Could you check a few things on this model? Use its own coordinates, in mm. A direction names the side the tool comes from. Coordinates: 2 decimals unless noted, no trailing zeros. Loops run counter-clockwise (first coordinate to the right, second up) from the corner with the lowest first, then second, coordinate; pieces in that order, holes last. Notation, with made-up numbers: (38.5, -7) -> (70.5, -7) arc R19 ccw to (70.5, 0) -> close; hole circle Ø1 at (19, -33.75). An arc over 180 degrees is marked (long way). One line per question, with ' | ' between items. Start each with the question number.
(1) If I drill on line 1 along Y through (x, z) = (0, 3.45); line 2 along X through (y, z) = (-32, 2.5); line 3 along Y through (x, z) = (-0.5, 9.25), over which ranges is the centre line in solid material (lowest first)?
(2) If we mould it in two halves opening along Z, with no side actions, what happens to faces 4 (the face through (4.95, -42.93, 8.72)), 5 (the face through (-0.581, 47.317, 16.797)), 6 (the face through (0.434, 27.548, 2.465))? For each: pulls with the +Z half, pulls with the -Z half, needs draft (parallel to the pull), parting line crosses it, or undercut.
(3) I'm going to push flat-ended pins straight in: pin 1 Ø4 at (y, z) = (-31.5, 8.5) entering from +X; pin 2 Ø1.2 at (x, y) = (0, 29.5) entering from -Z; pin 3 Ø0.8 at (x, z) = (0, 8.5) entering from -Y. Where does each tip first touch, or does it pass through?
(4) Suppose I cut it at A-A (x = 0). Please give me the cut outline in (y, z), plus the area to 3 significant figures.
(5) Which directions (+Z, -Z, +X, -X, +Y, -Y) give clear straight access to the entire face, cutting with the end or side of a thin tool? Please do faces 1 (the face through (0, 30, 5)), 2 (the face through (-46.3, 20, 8)), 3 (the face through (0, -43, 7.47)).
```python
from build123d import *

# Parameters (mm, degrees)
SKETCH1_W           = 93
SKETCH1_H           = 97
BOSS_EXTRUDE1_DEPTH = 17.5
FILLET1_SIZE        = 5
FILLET1_SIZE_2      = 10
FILLET2_SIZE        = 10
FILLET2_SIZE_2      = 5
FILLET3_SIZE        = 5
FILLET3_SIZE_2      = 10
SKETCH2_R           = 1.28
SKETCH2_W           = 7.34
SKETCH2_H           = 2.56
CUT_EXTRUDE1_DEPTH  = 11.3
SKETCH3_R           = 5
BOSS_EXTRUDE2_DEPTH = 0.6
CHAMFER1_SIZE       = 0.6
CUT_EXTRUDE2_DEPTH  = 0.2
CHAMFER4_SIZE       = 2.4
CHAMFER4_SIZE2      = 1.385640646
SKETCH5_R           = 2
CUT_EXTRUDE3_DEPTH  = 5


# Some blends are built 0.0001 mm under size
with BuildPart() as part:
    # Sketch1 → Boss-Extrude1 (new body)
    with BuildSketch(Plane.XY):
        Rectangle(SKETCH1_W, SKETCH1_H)
    extrude(amount=BOSS_EXTRUDE1_DEPTH)

    # Fillet1
    # an asymmetric fillet: 10, 5 mm, written as the material it takes off along each edge
    with BuildSketch(Plane(origin=(-46.5, 48.5, -25), x_dir=(1, 0, 0), z_dir=(0, 0, 1))) as fillet1_piece_1:
        with BuildLine():
            Bezier((FILLET1_SIZE, 0), (0, 0), (0, -FILLET1_SIZE_2), weights=[1, 0.707106781, 1])
            Line((0, -FILLET1_SIZE_2), (0, 0))
            Line((0, 0), (FILLET1_SIZE, 0))
        make_face()
    extrude(amount=67.5, mode=Mode.SUBTRACT)
    with BuildSketch(Plane(origin=(46.5, -48.5, -25), x_dir=(0, 1, 0), z_dir=(0, 0, 1))) as fillet1_piece_2:
        with BuildLine():
            Bezier((FILLET1_SIZE_2, 0), (0, 0), (0, FILLET1_SIZE), weights=[1, 0.707106781, 1])
            Line((0, FILLET1_SIZE), (0, 0))
            Line((0, 0), (FILLET1_SIZE_2, 0))
        make_face()
    extrude(amount=67.5, mode=Mode.SUBTRACT)

    # Fillet2
    # an asymmetric fillet: 10, 5 mm, written as the material it takes off along each edge
    with BuildSketch(Plane(origin=(-46.5, -48.5, -25), x_dir=(0, 1, 0), z_dir=(0, 0, 1))) as fillet2_piece_1:
        with BuildLine():
            Bezier((FILLET2_SIZE, 0), (0, 0), (0, -FILLET2_SIZE_2), weights=[1, 0.707106781, 1])
            Line((0, -FILLET2_SIZE_2), (0, 0))
            Line((0, 0), (FILLET2_SIZE, 0))
        make_face()
    extrude(amount=67.5, mode=Mode.SUBTRACT)

    # Fillet3
    # an asymmetric fillet: 10, 5 mm, written as the material it takes off along each edge
    with BuildSketch(Plane(origin=(46.5, 48.5, -25), x_dir=(-1, 0, 0), z_dir=(0, 0, 1))) as fillet3_piece_1:
        with BuildLine():
            Bezier((FILLET3_SIZE, 0), (0, 0), (0, FILLET3_SIZE_2), weights=[1, 0.707106781, 1])
            Line((0, FILLET3_SIZE_2), (0, 0))
            Line((0, 0), (FILLET3_SIZE, 0))
        make_face()
    extrude(amount=67.5, mode=Mode.SUBTRACT)

    # Sketch2 → Cut-Extrude1 (cut)
    with BuildSketch(Plane.XZ.offset(48.5)):
        with Locations((-3.67, 8.75)):
            Circle(SKETCH2_R)
        with Locations((3.67, 8.75)):
            Circle(SKETCH2_R)
        with Locations((0, 8.75)):
            Rectangle(SKETCH2_W, SKETCH2_H)
    extrude(amount=-CUT_EXTRUDE1_DEPTH, mode=Mode.SUBTRACT)

    # Sketch3 → Boss-Extrude2 (add)
    with BuildSketch(Plane(origin=(46.5, 0, 0), x_dir=(0, 0, -1), z_dir=(1, 0, 0))):
        with Locations(Location((-7.7, 8.5, 0), (0, 0, 270))):
            Circle(SKETCH3_R)
    extrude(amount=BOSS_EXTRUDE2_DEPTH)

    # Chamfer1
    chamfer1_edges = [part.edges().sort_by_distance(p)[0] for p in [
        (47.1, 13.5, 7.7),
    ]]
    chamfer(chamfer1_edges, length=CHAMFER1_SIZE - 0.0001)  # a hair under: the kernel refuses the full size

    # Sketch4 → Cut-Extrude2 (cut)
    with BuildSketch(Plane.ZY.offset(46.5)):
        with BuildLine():
            Line((3, 34.5), (13.7, 34.5))
            ThreePointArc((13.7, 34.5), (14.407106781, 34.207106781), (14.7, 33.5))
            Line((14.7, 33.5), (14.7, 6.8))
            ThreePointArc((14.7, 6.8), (14.407106781, 6.092893219), (13.7, 5.8))
            Line((13.7, 5.8), (3, 5.8))
            ThreePointArc((3, 5.8), (2.292893219, 6.092893219), (2, 6.8))
            Line((2, 6.8), (2, 33.5))
            ThreePointArc((2, 33.5), (2.292893219, 34.207106781), (3, 34.5))
        make_face()
    extrude(amount=-CUT_EXTRUDE2_DEPTH, mode=Mode.SUBTRACT)

    # Chamfer4
    chamfer4_edges = [part.edges().sort_by_distance(p)[0] for p in [
        (-45.520581957, 44.444718915, 17.5),
        (-46.5, 0, 17.5),
        (0, 48.5, 17.5),
        (-45.52058196, -44.444718917, 17.5),
        (45.520581957, 44.444718915, 17.5),
        (0, -48.5, 17.5),
        (46.5, 0, 17.5),
        (45.52058196, -44.444718917, 17.5),
    ]]
    chamfer4_side = [part.faces().sort_by_distance(p)[0] for p in [
        (0, 4.215e-06, 17.5),
    ]]
    chamfer(chamfer4_edges, length=CHAMFER4_SIZE, length2=CHAMFER4_SIZE2, reference=chamfer4_side[0])

    # Sketch5 → Cut-Extrude3 (cut)
    with BuildSketch(Plane(origin=(0, 0, 0), x_dir=(-1, 0, 0), z_dir=(0, 0, -1))):
        with Locations((0, 29.5)):
            Circle(SKETCH5_R)
    extrude(amount=-CUT_EXTRUDE3_DEPTH, mode=Mode.SUBTRACT)


solid = part.part
```
Checks:
1) line 1: y = -48.5 to 27.5, 31.5 to 48.5 | line 2: x = -46.5 to 46.5 | line 3: y = -37.2 to 48.5
2) face 4: undercut | face 5: pulls with the +Z half | face 6: needs draft
3) pin 1: stops at x = 46.5 | pin 2: stops at z = 5 | pin 3: stops at y = -37.2
4) outline: (-48.5, 0) -> (27.5, 0) -> (27.5, 5) -> (31.5, 5) -> (31.5, 0) -> (48.5, 0) -> (48.5, 16.11) -> (46.1, 17.5) -> (-46.1, 17.5) -> (-48.5, 16.11) -> (-48.5, 10.03) -> (-37.2, 10.03) -> (-37.2, 7.47) -> (-48.5, 7.47) -> close | area: 1,650 mm^2
5) face 1: -Z | face 2: -X | face 3: -Y
